```python
from build123d import *

# Parameters (mm, degrees)
SKETCH1_W           = 1117.6
SKETCH1_H           = 1219.2
BOSS_EXTRUDE1_DEPTH = 6.35
SKETCH2_W           = 6.35
SKETCH2_H           = 1219.2
BOSS_EXTRUDE2_DEPTH = 50.8
FILLET1_R           = 5


with BuildPart() as part:
    # Sketch1 → Boss-Extrude1 (new body)
    with BuildSketch(Plane.XY):
        with Locations((558.8, 609.6)):
            Rectangle(SKETCH1_W, SKETCH1_H)
    extrude(amount=BOSS_EXTRUDE1_DEPTH)

    # Sketch2 → Boss-Extrude2 (add)
    with BuildSketch(Plane.XY.offset(6.35)):
        with Locations((3.175, 609.6)):
            Rectangle(SKETCH2_W, SKETCH2_H)
        with Locations((1114.425, 609.6)):
            Rectangle(SKETCH2_W, SKETCH2_H)
    extrude(amount=BOSS_EXTRUDE2_DEPTH)

    # Fillet1
    fillet1_edges = [part.edges().sort_by_distance(p)[0] for p in [
        (6.35, 609.6, 6.35),
        (1111.25, 609.6, 6.35),
        (1117.6, 609.6, 0),
        (0, 609.6, 0),
    ]]
    fillet(fillet1_edges, radius=FILLET1_R)


solid = part.part
```
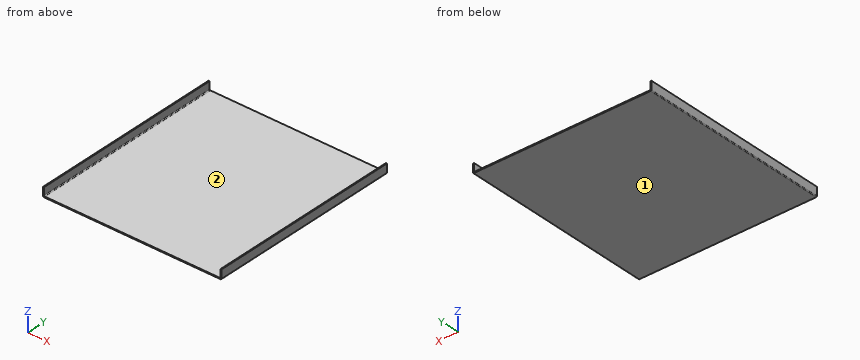
Check sheet for the modelled part. Datum: model origin and axes. Units: mm. Face numbers are marked on the shaded views. Round coordinates to 2 decimals unless told otherwise and drop trailing zeros. Write each loop counter-clockwise with the first axis right and the second up, starting at its lowest first coordinate (ties: lowest second). Pieces come first, ordered by that corner, then holes. Notation, with made-up numbers: (0, 24.5) -> (33, 24.5) arc R26 cw to (33, 45.5) -> close; hole circle Ø5 at (64, -5.75). An arc over 180 degrees is marked (long way). Put each result on its own line as item: value.
(1) Sectioned sample at C-C (x = 590.5). Enter the section's corners in (y, z).
Values found:
outline: (0, 0) -> (1219.2, 0) -> (1219.2, 6.35) -> (0, 6.35) -> close
(2) Sectioned sample at B-B (y = 276). Enter the section's corners in (x, z).
Values found:
outline: (0, 5) arc R5 ccw to (5, 0) -> (1112.6, 0) arc R5 ccw to (1117.6, 5) -> (1117.6, 57.15) -> (1111.25, 57.15) -> (1111.25, 11.35) arc R5 cw to (1106.25, 6.35) -> (11.35, 6.35) arc R5 cw to (6.35, 11.35) -> (6.35, 57.15) -> (0, 57.15) -> close
(3) Material ranges on line 1 (X direction, y = 818, z = 36); line 2 (Z direction, x = 188, y = 767.5); line 3 (X direction, y = 940, z = 8.5), recorded low to high.
Values found:
line 1: x = 0 to 6.35, 1111.25 to 1117.6
line 2: z = 0 to 6.35
line 3: x = 0 to 7.24, 1110.36 to 1117.6
(4) Go/stop test with flat-tipped pins: pin 1 Ø12 at (x, z) = (184.5, 14) entering from +Y; pin 2 Ø2 at (x, y) = (286, 972.5) entering from +Z. Record where each tip stops, or that it passes through.
Values found:
pin 1: passes through
pin 2: stops at z = 6.35
(5) Sectioned sample at A-A (z = 36.5). Enter the section's corners in (x, y), plus the area to 3 significant figures.
Values found:
outline: (0, 0) -> (6.35, 0) -> (6.35, 1219.2) -> (0, 1219.2) -> close; (1111.25, 0) -> (1117.6, 0) -> (1117.6, 1219.2) -> (1111.25, 1219.2) -> close
area: 15,500 mm^2
(6) Mould release check, pull along X, two halves, no side actions. Record for the marked faces 1 and 2: released by +X, released by -X, zero draft, split by the parting line, or undercut.
Values found:
face 1: zero draft
face 2: undercut
